Here's how the part is built. I have some questions about the finished solid (model axes, mm). Give positions to 0.01 mm unless a question says otherwise; leave off trailing zeros. Order: outer loops, then holes, each group sorted by start corner. A loop starts at its lowest first (then second) coordinate and runs counter-clockwise, first axis right, second up. Notation, with made-up numbers: M -17.75,39.25 L 24.25,39.25 A10 cw 24.25,57.25 Z; hole C 8.25,-38 d9. An arc over 180 degrees is marked long. Use one line per item in the form item = value.
from build123d import *

# Parameters (mm, degrees)
SKETCH1_W           = 101.5
SKETCH1_H           = 23
BOSS_EXTRUDE1_DEPTH = 2.8
SKETCH2_W           = 3
SKETCH2_H           = 1
CUT_EXTRUDE1_DEPTH  = 33
SKETCH3_W           = 3
SKETCH3_H           = 1
CUT_EXTRUDE2_DEPTH  = 33


with BuildPart() as part:
    # Sketch1 → Boss-Extrude1 (new body)
    with BuildSketch(Plane.XY):
        with Locations((50.75, 11.5)):
            Rectangle(SKETCH1_W, SKETCH1_H)
    extrude(amount=BOSS_EXTRUDE1_DEPTH)

    # Sketch2 → Cut-Extrude1 (cut)
    with BuildSketch(Plane(origin=(0, 23, 0), x_dir=(1, 0, 0), z_dir=(0, 1, 0))):
        with Locations((50.75, -0.5)):
            Rectangle(SKETCH2_W, SKETCH2_H)
    extrude(amount=-CUT_EXTRUDE1_DEPTH, mode=Mode.SUBTRACT)

    # Sketch3 → Cut-Extrude2 (cut)
    with BuildSketch(Plane(origin=(0, 23, 0), x_dir=(1, 0, 0), z_dir=(0, 1, 0))):
        with Locations((50.75, -2.3)):
            Rectangle(SKETCH3_W, SKETCH3_H)
    extrude(amount=-CUT_EXTRUDE2_DEPTH, mode=Mode.SUBTRACT)


solid = part.part
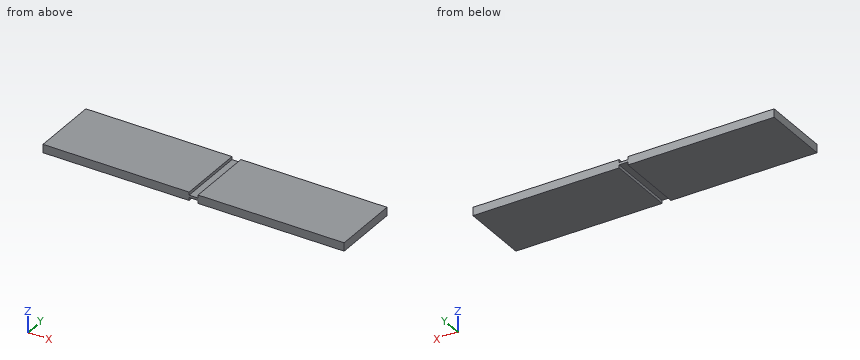
Q1. I need wall thicknesses on L1, parallel to X at y = 15.5, z = 0.65. Which ranges of the line are inside material? Lowest first, please.
Found:
L1 = 0 to 49.25, 52.25 to 101.5
Q2. I'm going to push a flat-ended pin straight in: pin 1 Ø10 at (x, y) = (76, 7) entering from -Z. Where does the tip first touch, or does it pass through?
Found:
pin_1 = 0
Q3. I want a section at B-B on y = 7.5. Write out the boundary of the cut face in (x, z), then the cut area to 3 significant figures.
Found:
outline = M 0,0 L 49.25,0 L 49.25,1 L 52.25,1 L 52.25,0 L 101.5,0 L 101.5,2.8 L 52.25,2.8 L 52.25,1.8 L 49.25,1.8 L 49.25,2.8 L 0,2.8 Z
area = 278 mm²
Q4. I want a section at A-A on z = 0.5. Write out the boundary of the cut face in (x, y).
Found:
outline = M 0,0 L 49.25,0 L 49.25,23 L 0,23 Z; M 52.25,0 L 101.5,0 L 101.5,23 L 52.25,23 Z
